The listing builds one solid part. Answer for the finished solid, in the listing's coordinates (mm). Give positions to 0.01 mm unless a question says otherwise; leave off trailing zeros. Write each loop counter-clockwise with the first axis right and the second up, starting at its lowest first coordinate (ties: lowest second). Pieces come first, ordered by that corner, then holes.
```python
from build123d import *

# Parameters (mm, degrees)
SKETCH1_W           = 43.18
SKETCH1_H           = 58.42
BOSS_EXTRUDE1_DEPTH = 1.5875
BOSS_EXTRUDE2_DEPTH = 0.1


with BuildPart() as part:
    # Sketch1 → Boss-Extrude1 (new body)
    with BuildSketch(Plane(origin=(0, 0, 0), x_dir=(1, 0, 0), z_dir=(0, 1, 0))):
        with Locations((21.59, 29.21)):
            Rectangle(SKETCH1_W, SKETCH1_H)
    extrude(amount=BOSS_EXTRUDE1_DEPTH)

    # Sketch2 → Boss-Extrude2 (add)
    with BuildSketch(Plane(origin=(0, 1.5875, 0), x_dir=(1, 0, 0), z_dir=(0, 1, 0))):
        Polygon((2.217, 7.24), (41.38, 7.24), (41.38, 5.91), (39.746, 5.91), (39.746, 0.25), (38.526, 0.25), (38.526, 5.91), (37.688, 5.91), (37.688, 0.25), (36.468, 0.25), (36.468, 5.91), (35.63, 5.91), (35.63, 0.25), (34.41, 0.25), (34.41, 5.91), (33.572, 5.91), (33.572, 0.25), (32.352, 0.25), (32.352, 5.91), (31.514, 5.91), (31.514, 0.25), (30.294, 0.25), (30.294, 5.91), (29.456, 5.91), (29.456, 0.25), (28.236, 0.25), (28.236, 5.91), (27.398, 5.91), (27.398, 0.25), (26.178, 0.25), (26.178, 5.91), (25.34, 5.91), (25.34, 0.25), (24.12, 0.25), (24.12, 5.91), (23.282, 5.91), (23.282, 0.25), (22.062, 0.25), (22.062, 5.91), (21.224, 5.91), (21.224, 0.25), (20.004, 0.25), (20.004, 5.91), (19.166, 5.91), (19.166, 0.25), (17.946, 0.25), (17.946, 5.91), (17.108, 5.91), (17.108, 0.25), (15.888, 0.25), (15.888, 5.91), (15.05, 5.91), (15.05, 0.25), (13.83, 0.25), (13.83, 5.91), (12.992, 5.91), (12.992, 0.25), (11.772, 0.25), (11.772, 5.91), (10.934, 5.91), (10.934, 0.25), (9.714, 0.25), (9.714, 5.91), (8.876, 5.91), (8.876, 0.25), (7.656, 0.25), (7.656, 5.91), (6.818, 5.91), (6.818, 0.25), (5.598, 0.25), (5.598, 5.91), (4.76, 5.91), (4.76, 0.25), (3.54, 0.25), (3.54, 5.91), (2.217, 5.91), align=None)
        Polygon((41.38, 53), (2.217, 53), (2.217, 54.33), (3.54, 54.33), (3.54, 58.17), (4.76, 58.17), (4.76, 54.33), (5.598, 54.33), (5.598, 58.17), (6.818, 58.17), (6.818, 54.33), (7.656, 54.33), (7.656, 58.17), (8.876, 58.17), (8.876, 54.33), (9.714, 54.33), (9.714, 58.17), (10.934, 58.17), (10.934, 54.33), (11.772, 54.33), (11.772, 58.17), (12.992, 58.17), (12.992, 54.33), (13.83, 54.33), (13.83, 58.17), (15.05, 58.17), (15.05, 54.33), (15.888, 54.33), (15.888, 58.17), (17.108, 58.17), (17.108, 54.33), (17.946, 54.33), (17.946, 58.17), (19.166, 58.17), (19.166, 54.33), (20.004, 54.33), (20.004, 58.17), (21.224, 58.17), (21.224, 54.33), (22.062, 54.33), (22.062, 58.17), (23.282, 58.17), (23.282, 54.33), (24.12, 54.33), (24.12, 58.17), (25.34, 58.17), (25.34, 54.33), (26.178, 54.33), (26.178, 58.17), (27.398, 58.17), (27.398, 54.33), (28.236, 54.33), (28.236, 58.17), (29.456, 58.17), (29.456, 54.33), (30.294, 54.33), (30.294, 58.17), (31.514, 58.17), (31.514, 54.33), (32.352, 54.33), (32.352, 58.17), (33.572, 58.17), (33.572, 54.33), (34.41, 54.33), (34.41, 58.17), (35.63, 58.17), (35.63, 54.33), (36.468, 54.33), (36.468, 58.17), (37.688, 58.17), (37.688, 54.33), (38.526, 54.33), (38.526, 58.17), (39.746, 58.17), (39.746, 54.33), (41.38, 54.33), align=None)
    extrude(amount=BOSS_EXTRUDE2_DEPTH)


solid = part.part
```
Item 1: A cutting plane is placed at A-A, the plane z = -52. Give the vertices of the cut face in (x, y), plus the area to 3 significant figures.
Conclusion:
outline: (0, 0) - (43.18, 0) - (43.18, 1.59) - (0, 1.59) - close
area: 68.5 mm2
Item 2: Consider probe 1 along Y at (x, z) = (8, -19). Determine where the line is inside the solid, lowest interval first.
Conclusion:
probe 1: y = 0 to 1.59
Item 3: Determine the mould class of faces 1 (the face through (21, 1.588, -30)), 2 (the face through (21, 0, -30)), 3 (the face through (21, 1, -58.42)) for opening direction Z: pulls with the +Z half, pulls with the -Z half, needs draft (parallel to the pull), parting line crosses it, or undercut.
Conclusion:
face 1: undercut
face 2: needs draft
face 3: pulls with the -Z half
